Geometry: final body of the model. Coordinates: model frame, mm. A direction names the side the tool comes from. Give positions to 0.01 mm unless a question says otherwise; leave off trailing zeros. Write each loop counter-clockwise with the first axis right and the second up, starting at its lowest first coordinate (ties: lowest second). Pieces come first, ordered by that corner, then holes. Notation, with made-up numbers: (84.25, -39) -> (125.25, -39) arc R11 cw to (125.25, -25) -> close; hole circle Ø8 at (11, 19). An arc over 180 degrees is marked (long way). Answer as a JSON object with one key per item and string values.
from build123d import *

# Parameters (mm, degrees)
F1_DEPTH = 8.128
F0_W     = 10.668
F0_H     = 65.8876
F0_W_2   = 8.382
F0_H_2   = 6.35
F2_DEPTH = 25.4
F3_W     = 10.668
F3_H     = 3.302
F4_DEPTH = 0.762
F5_W     = 19.05
F5_H     = 3.302
F6_DEPTH = 0.762


# Not quite as in the source:
# - a feature names something its author has since deleted; it is built from what else it names


with BuildPart() as f1:
    # F0 (on Top) → F1 (new body)
    with BuildSketch(Plane.XY):
        Polygon((18.4785, -32.9438), (18.4785, 32.9438), (-1.905, 32.9438), (-18.4785, 32.9438), (-18.4785, -32.9438), (-9.652, -32.9438), (9.652, -32.9438), align=None)
    extrude(amount=F1_DEPTH)

    # F0 (on Top) → F2 (join)
    with BuildSketch(Plane.XY):
        with Locations((-23.8125, 0)):
            Rectangle(F0_W, F0_H)
        with Locations((33.3375, 29.7688)):
            Rectangle(F0_W_2, F0_H_2)
        Polygon((29.1465, 26.5938), (29.1465, 32.9438), (18.4785, 32.9438), (18.4785, -32.9438), (29.1465, -32.9438), (29.1465, -20.2438), align=None)
    extrude(amount=F2_DEPTH)

    # F3 (on face) → F4 (cut)
    with BuildSketch(Plane.XZ.offset(32.9438)):
        with Locations((23.8125, 13.843)):
            Rectangle(F3_W, F3_H)
        with Locations((23.8125, 20.828)):
            Rectangle(F3_W, F3_H)
    extrude(amount=-F4_DEPTH, mode=Mode.SUBTRACT)

    # F5 (on face) → F6 (cut)
    with BuildSketch(Plane(origin=(0, 32.9438, 0), x_dir=(-1, 0, 0), z_dir=(0, 1, 0))):
        with Locations((-28.0035, 17.3482)):
            Rectangle(F5_W, F5_H)
    extrude(amount=-F6_DEPTH, mode=Mode.SUBTRACT)


solid = f1.part
Q1. Cut plane D-D (z = 3.25). Return the cut outline in (x, y), and give its area (3 significant figures).
Values:
{"outline": "(-29.15, -32.94) -> (29.15, -32.94) -> (29.15, 26.59) -> (37.53, 26.59) -> (37.53, 32.94) -> (-29.15, 32.94) -> close", "area": "3,890 mm²"}
Q2. Cut plane C-C (z = 18). Return the cut outline in (x, y).
Values:
{"outline": "(-29.15, -32.94) -> (-18.48, -32.94) -> (-18.48, 32.94) -> (-29.15, 32.94) -> close; (18.48, -32.94) -> (29.15, -32.94) -> (29.15, 26.59) -> (37.53, 26.59) -> (37.53, 32.18) -> (18.48, 32.18) -> close"}
Q3. Cut plane A-A (z = 10.75). Return the cut outline in (x, y).
Values:
{"outline": "(-29.15, -32.94) -> (-18.48, -32.94) -> (-18.48, 32.94) -> (-29.15, 32.94) -> close; (18.48, -32.94) -> (29.15, -32.94) -> (29.15, 26.59) -> (37.53, 26.59) -> (37.53, 32.94) -> (18.48, 32.94) -> close"}
Q4. Mould query, pull axis Z, two halves, no side actions, for faces 6 (the flat face through (-24, 0, 25.4)), 7 (the flat face through (28, 32.944, 22)), 8 (the flat face through (24, -32.182, 21)). Classes: pulls with the +Z half, pulls with the -Z half, needs draft (parallel to the pull), parting line crosses it, or undercut.
Values:
{"face 6": "pulls with the +Z half", "face 7": "needs draft", "face 8": "undercut"}
Q5. Cut plane B-B (y = -12). Return the cut outline in (x, z).
Values:
{"outline": "(-29.15, 0) -> (29.15, 0) -> (29.15, 25.4) -> (18.48, 25.4) -> (18.48, 8.13) -> (-18.48, 8.13) -> (-18.48, 25.4) -> (-29.15, 25.4) -> close"}
Q6. Material intervals for L1, parallel to X at y = 22.5, z = 17.25; L2, parallel to Y at x = 30, z = 7.5; L3, parallel to Z at x = 0, y = -27, sorted ascending. Write a range as from..to.
Values:
{"L1": "-29.15..-18.48, 18.48..29.15", "L2": "26.59..32.94", "L3": "0..8.13"}
Q7. Set-up query: faces 1 (the flat face through (-7, -32.944, 7)), 2 (the flat face through (28, 32.182, 17)), 3 (the flat face through (24, -32.182, 14)), 4 (the flat face through (18.478, 0, 17)), 5 (the flat face through (33, 26.594, 13)). Return all of +Z, -Z, +X, -X, +Y, -Y with unobstructed straight access to the full face (end or side cutting, diameter ignored); none if empty.
Values:
{"face 1": "+Z, -Z, +X, -X, -Y", "face 2": "+X, +Y", "face 3": "+X, -Y", "face 4": "+Z, +Y, -Y", "face 5": "+Z, -Z, +X, -Y"}
Q8. First-contact query: P1, Ø1, axis at x = 25, z = 14.5, coming from the -Y side; P2, Ø1.7, axis at x = 26.5, z = 18, coming from the +Y side; P3, Ø0.6, axis at x = 29.5, y = 32.5, coming from the -Z side; P4, Ø2, axis at y = 12.5, z = 7.5, coming from the +X side. Flat tips, straight axial feed; report the tip coordinate or a pass-through.
Values:
{"P1": "y = -32.18", "P2": "y = 32.18", "P3": "z = 0", "P4": "x = 29.15"}
